Verification items for this drawing (mm, ordinates from the low corner). A direction names the side the tool comes from. Give positions to 0.01 mm unless a question says otherwise; leave off trailing zeros. Loops run counter-clockwise (first coordinate to the right, second up) from the corner with the lowest first, then second, coordinate; pieces in that order, holes last. Notation, with made-up numbers: M 82.5,-11.75 L 98.5,-11.75 A26 cw 98.5,25.25 Z; hole C -27.5,87 d9. An arc over 180 degrees is marked long. Answer in a Markdown table with one row per item.
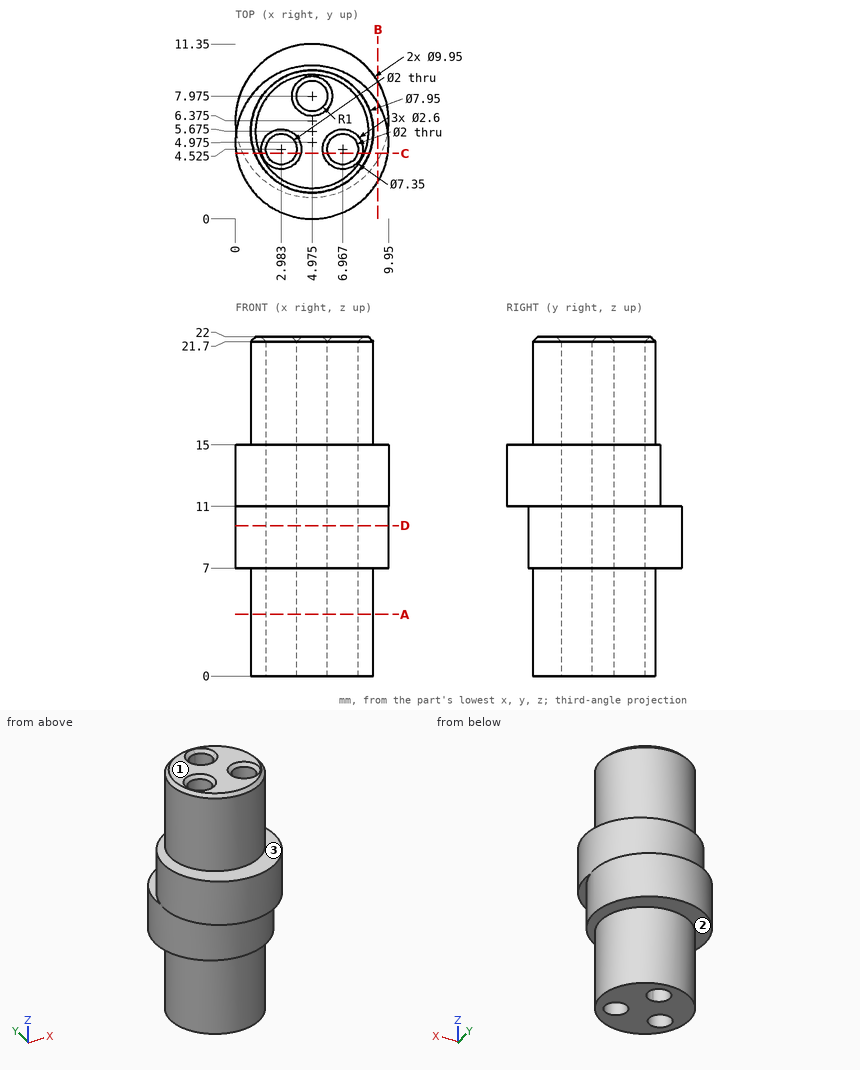
Item 1: Sectioned sample at B-B (x = 9.25). Record the cut outline in (y, z), and give its area (3 significant figures).
Reported:
| item | result |
|---|---|
| outline | M 2.43,11 L 3.83,11 L 3.83,7 L 8.92,7 L 8.92,11 L 7.52,11 L 7.52,15 L 2.43,15 Z |
| area | 40.7 mm^2 |
Item 2: Tool access check on the marked faces 1, 2 and 3. Record the directions out of +Z, -Z, +X, -X, +Y, -Y that give a thin tool (end or side, any length) a straight path to the whole face; none if there is none.
Reported:
| item | result |
|---|---|
| face 1 | +Z, +X, -X, +Y, -Y |
| face 2 | -Z |
| face 3 | +Z |
Item 3: Scan lines: L1, parallel to X at y = 4.25, z = 13.25 (1 decimal); L2, parallel to X at y = 5.25, z = 1.75 (1 decimal); L3, parallel to X at y = 1.25, z = 12.75. Record each from-to range of solid material in increasing order. Write a range as [from, to].
Reported:
| item | result |
|---|---|
| L1 | x = [0.1, 2], [3.9, 6], [7.9, 9.9] |
| L2 | x = [1, 2.3], [3.7, 6.3], [7.7, 8.9] |
| L3 | x = [1.68, 8.27] |
Item 4: Sectioned sample at A-A (z = 4). Record the cut outline in (x, y) (3 decimals).
Reported:
| item | result |
|---|---|
| outline | C 4.975,5.675 d7.95; hole C 2.983,4.525 d2; hole C 4.975,7.975 d2; hole C 6.967,4.525 d2 |
Item 5: Go/stop test with flat-tipped pins: pin 1 (2 mm diameter, centred on x = 5, z = 4.5, fed in from -Y); pin 2 (1.7 mm diameter, centred on x = 4.5, y = 2.5, fed in from -Z); pin 3 (2 mm diameter, centred on x = 1.5, z = 11.5, fed in from +Y); pin 4 (2 mm diameter, centred on x = 3, z = 13, fed in from -Y). Record where each tip stops, or that it passes through.
Reported:
| item | result |
|---|---|
| pin 1 | stops at y = 1.7 |
| pin 2 | stops at z = 0 |
| pin 3 | stops at y = 10.61 |
| pin 4 | stops at y = 0.1 |
Item 6: Sectioned sample at D-D (z = 9.75). Record the cut outline in (x, y) (3 decimals), and give its area (3 significant figures).
Reported:
| item | result |
|---|---|
| outline | C 4.975,6.375 d9.95; hole C 2.983,4.525 d2; hole C 4.975,7.975 d2; hole C 6.967,4.525 d2 |
| area | 68.3 mm^2 |
Item 7: Sectioned sample at C-C (y = 4.25). State how many separate pieces and enclosed holes the cut face has.
Reported:
| item | result |
|---|---|
| separate pieces | 3 |
| enclosed holes | 0 |
